For this review, use the dimensioned drawing (mm, ordinates from the lowest corner) and the shaded views. A direction names the side the tool comes from. Give positions to 0.01 mm unless a question says otherwise; leave off trailing zeros. Loops run counter-clockwise (first coordinate to the right, second up) from the corner with the lowest first, then second, coordinate; pieces in that order, holes last. Notation, with made-up numbers: (44, -16.5) -> (51, -16.5) arc R9 ccw to (51, 0.5) -> close; hole circle Ø3 at (7.5, -2.5). An arc over 180 degrees is marked (long way). Write each question's results on one line, items separated by ' | '. Start each with the question number.
Q1. Mouldability with a two-part tool opening along Y and no side actions: class the marked faces 1, 2, 3 and 4 as released by +Y, released by -Y, zero draft, split by the parting line, or undercut.
Q2. We need section B-B (x = 38.5). Write out the cut boundary in (y, z), plus the area to 3 significant figures.
Q3. Machinability: for the marked faces 5 and 6, which of the approach directions +Z, -Z, +X, -X, +Y, -Y give a long, thin tool a straight path to every point of the face, cutting with its end or side? Answer none if there is none.
Q4. Insertion check: pin 1 Ø10 at (x, y) = (87, 56.5) entering from -Z; pin 2 Ø12.5 at (y, z) = (64, 59.5) entering from +X; pin 3 Ø8 at (x, y) = (64.5, 21) entering from +Z; pin 4 Ø13.5 at (x, z) = (40.5, 60) entering from +Y. Each pin has a flat end and moves straight along its axis. Give the tip position at first contact, or say it passes through.
Q5. We need section C-C (y = 32.5). Write out the cut boundary in (x, z).
Q6. Wall thickness on L1, parallel to Z at x = 97, y = 121.5; L2, parallel to Y at x = 38, z = 59; L3, parallel to Z at x = 62, y = 79 (1 decimal): over which ranges is each line inside the solid? List them lowest first. Write a range as [from, to].
Q7. We need section D-D (z = 62.5). Write out the cut boundary in (x, y).
Q8. We need section A-A (z = 49). Write out the cut boundary in (x, y), plus the area to 3 significant figures.
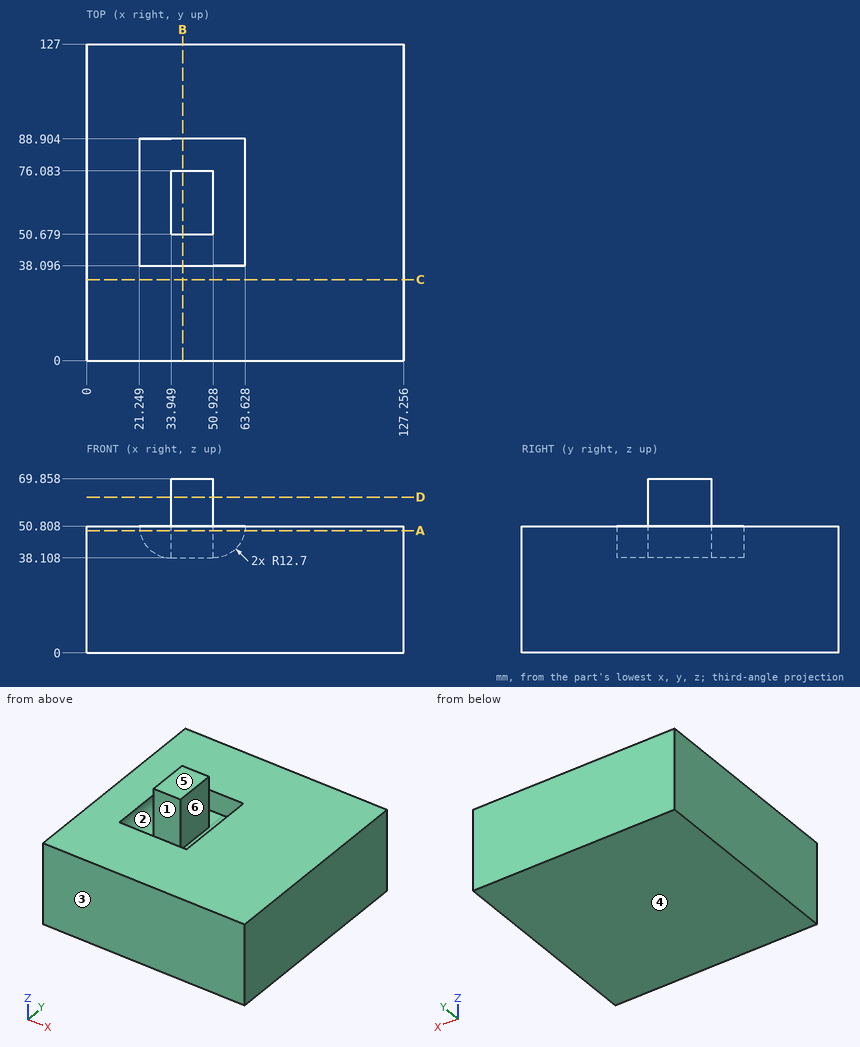
Output:
1) face 1: undercut | face 2: undercut | face 3: released by -Y | face 4: zero draft
2) outline: (0, 0) -> (127, 0) -> (127, 50.81) -> (88.9, 50.81) -> (88.9, 38.11) -> (76.08, 38.11) -> (76.08, 69.86) -> (50.68, 69.86) -> (50.68, 38.11) -> (38.1, 38.11) -> (38.1, 50.81) -> (0, 50.81) -> close | area: 6,610 mm2
3) face 5: +Z, +X, -X, +Y, -Y | face 6: +Z
4) pin 1: z = 0 | pin 2: x = 50.93 | pin 3: z = 50.81 | pin 4: y = 76.08
5) outline: (0, 0) -> (127.26, 0) -> (127.26, 50.81) -> (0, 50.81) -> close
6) L1: [0, 50.81] | L2: [50.68, 76.08] | L3: [0, 44.6]
7) outline: (33.95, 50.68) -> (50.93, 50.68) -> (50.93, 76.08) -> (33.95, 76.08) -> close
8) outline: (0, 0) -> (127.26, 0) -> (127.26, 127) -> (0, 127) -> close; (33.95, 50.68) -> (50.93, 50.68) -> (50.93, 76.08) -> (33.95, 76.08) -> close; hole (21.38, 38.1) -> (63.5, 38.1) -> (63.5, 88.9) -> (21.38, 88.9) -> close | area: 14,500 mm2
